Verification items for the finished model (mm, model axes). A direction names the side the tool comes from. Coordinates: 2 decimals unless noted, no trailing zeros. Write each loop counter-clockwise with the first axis right and the second up, starting at its lowest first coordinate (ties: lowest second). Pieces come first, ordered by that corner, then holes. Notation, with made-up numbers: (50.25, 36) - (73.25, 36) arc R27 ccw to (73.25, 71) - close; hole circle Ø4 at (39.25, 78.25). An arc over 180 degrees is marked (long way). Answer as CSV lines item,"result". Start each with the question number.
```python
from build123d import *

# Parameters (mm, degrees)
ESQUISSE1_W             = 10
ESQUISSE1_H             = 10
BOSS_EXTRU_1_DEPTH      = 10
ESQUISSE2_R             = 1.5
ENL_V_MAT_EXTRU_1_DEPTH = 11
ESQUISSE3_R             = 3
ENL_V_MAT_EXTRU_2_DEPTH = 8
ESQUISSE4_R             = 1.5
ENL_V_MAT_EXTRU_3_DEPTH = 11
ESQUISSE5_R             = 3
ENL_V_MAT_EXTRU_4_DEPTH = 8
ESQUISSE6_R             = 1.5
ENL_V_MAT_EXTRU_5_DEPTH = 11
ESQUISSE7_R             = 3
ENL_V_MAT_EXTRU_6_DEPTH = 8


with BuildPart() as part:
    # Esquisse1 → Boss.-Extru.1 (new body)
    with BuildSketch(Plane.XY):
        with Locations((5, 5)):
            Rectangle(ESQUISSE1_W, ESQUISSE1_H)
    extrude(amount=BOSS_EXTRU_1_DEPTH)

    # Esquisse2 → Enlèv. mat.-Extru.1 (cut, through all)
    with BuildSketch(Plane.XY.offset(10)):
        with Locations((5, 5)):
            Circle(ESQUISSE2_R)
    extrude(amount=-ENL_V_MAT_EXTRU_1_DEPTH, mode=Mode.SUBTRACT)

    # Esquisse3 → Enlèv. mat.-Extru.2 (cut)
    with BuildSketch(Plane.XY.offset(10)):
        with Locations((5, 5)):
            Circle(ESQUISSE3_R)
    extrude(amount=-ENL_V_MAT_EXTRU_2_DEPTH, mode=Mode.SUBTRACT)

    # Esquisse4 → Enlèv. mat.-Extru.3 (cut, through all)
    with BuildSketch(Plane(origin=(10, 0, 0), x_dir=(0, 0, -1), z_dir=(1, 0, 0))):
        with Locations((-5, 5)):
            Circle(ESQUISSE4_R)
    extrude(amount=-ENL_V_MAT_EXTRU_3_DEPTH, mode=Mode.SUBTRACT)

    # Esquisse5 → Enlèv. mat.-Extru.4 (cut)
    with BuildSketch(Plane(origin=(10, 0, 0), x_dir=(0, 0, -1), z_dir=(1, 0, 0))):
        with Locations((-5, 5)):
            Circle(ESQUISSE5_R)
    extrude(amount=-ENL_V_MAT_EXTRU_4_DEPTH, mode=Mode.SUBTRACT)

    # Esquisse6 → Enlèv. mat.-Extru.5 (cut, through all)
    with BuildSketch(Plane.XZ):
        with Locations((5, 5)):
            Circle(ESQUISSE6_R)
    extrude(amount=-ENL_V_MAT_EXTRU_5_DEPTH, mode=Mode.SUBTRACT)

    # Esquisse7 → Enlèv. mat.-Extru.6 (cut)
    with BuildSketch(Plane(origin=(0, 0, 0), x_dir=(-1, 0, 0), z_dir=(0, -1, 0))):
        with Locations((-5, -5)):
            Circle(ESQUISSE7_R)
    extrude(amount=-ENL_V_MAT_EXTRU_6_DEPTH, mode=Mode.SUBTRACT)


solid = part.part
```
1. Draft check along Y on faces 5 (the face through (2.7, 0, 2.7)), 6 (the face through (7.13, 7.11, 2.28)), 7 (the face through (10, 2.7, 2.7)). Enter one of: pulls with the +Y half, pulls with the -Y half, needs draft (parallel to the pull), parting line crosses it, or undercut.
2. Depth check by flat-ended pin: P1, Ø1.8, axis at x = 5, z = 6, coming from the -Y side; P2, Ø3, axis at x = 4.5, y = 6, coming from the +Z side; P3, Ø3.5, axis at y = 5, z = 5, coming from the +X side; P4, Ø2.5, axis at x = 5, y = 5, coming from the +Z side. Enter the tip coordinate at first touch or a pass-through.
3. Cross-section at B-B (x = 7.75). Record the cut outline in (y, z).
4. Cross-section at A-A (z = 7.5). Record the cut outline in (x, y).
5. Cross-section at C-C (x = 0.75). Record the cut outline in (y, z), and give its area (3 significant figures).
6. Scan lines: line 1 along Y through (x, z) = (5, 9.3); line 2 along Y through (x, z) = (2.75, 5.75). Record each from-to range of solid material in increasing order. Write a range as from..to.
7. Access from +Z, -Z, +X, -X, +Y, -Y to the whole of each face (thin tool, end or side, straight path). Record for faces 1 (the face through (2.28, 2.87, 2.89)), 2 (the face through (7.11, 2.87, 2.28)), 3 (the face through (6.386, 4.425, 1.014)), 4 (the face through (7.11, 7.72, 2.87)).
8. Cross-section at D-D (z = 8.5). Record the cut outline in (x, y).
Completed:
1,face 5,"pulls with the -Y half"
1,face 6,"undercut"
1,face 7,"needs draft"
2,P1,"stops at y = 8"
2,P2,"stops at z = 2"
2,P3,"stops at x = 2"
2,P4,"passes through"
3,outline,"(0, 0) - (10, 0) - (10, 10) - (6.2, 10) - (6.2, 7.75) arc R3 cw to (7.75, 6.2) - (8, 6.2) - (8, 3.8) - (7.75, 3.8) arc R3 cw to (6.2, 2.25) - (6.2, 2) - (3.8, 2) - (3.8, 2.25) arc R3 cw to (2.25, 3.8) - (0, 3.8) - close; (0, 6.2) - (2.25, 6.2) arc R3 cw to (3.8, 7.75) - (3.8, 10) - (0, 10) - close"
4,outline,"(0, 0) - (3.34, 0) - (3.34, 2.5) arc R3 cw to (2.5, 3.34) - (2, 3.34) - (2, 6.66) - (2.5, 6.66) arc R3 cw to (3.34, 7.5) - (3.34, 8) - (6.66, 8) - (6.66, 7.5) arc R3 cw to (7.5, 6.66) - (10, 6.66) - (10, 10) - (0, 10) - close; (6.66, 0) - (10, 0) - (10, 3.34) - (7.5, 3.34) arc R3 cw to (6.66, 2.5) - close"
5,outline,"(0, 0) - (10, 0) - (10, 10) - (0, 10) - close; hole circle Ø3 at (5, 5)"
5,area,"92.9 mm2"
6,line 1,"y = 0..2, 8..10"
6,line 2,"y = 8..10"
7,face 1,"+X"
7,face 2,"+Z"
7,face 3,"+Z, -Z"
7,face 4,"-Y"
8,outline,"(0, 0) - (10, 0) - (10, 10) - (0, 10) - close; hole circle Ø6 at (5, 5)"
